from build123d import *

# Parameters (mm, degrees)
CYLINDER062_R       = 1.8
CYLINDER062_DEPTH   = 12
ARRAY001032_X_COUNT = 2
ARRAY001032_X_PITCH = 76
ARRAY001032_Y_COUNT = 2
ARRAY001032_Y_PITCH = 26
BOX036_W            = 4
BOX036_H            = 50
BOX036_DEPTH        = 10
FILLET018_R         = 1
ARRAY001038_X_COUNT = 2
ARRAY001038_X_PITCH = 58
CYLINDER064_R       = 3
CYLINDER064_DEPTH   = 12
ARRAY001034_X_COUNT = 2
ARRAY001034_X_PITCH = 76
ARRAY001034_Y_COUNT = 2
ARRAY001034_Y_PITCH = 26
CYLINDER063_R       = 5
CYLINDER063_DEPTH   = 10
ARRAY001033_X_COUNT = 2
ARRAY001033_X_PITCH = 76
ARRAY001033_Y_COUNT = 2
ARRAY001033_Y_PITCH = 26
CYLINDER066_R       = 1.8
CYLINDER066_DEPTH   = 50
ARRAY001036_Y_COUNT = 4
ARRAY001036_Y_PITCH = 6
BOX033_W            = 36
BOX033_H            = 25
BOX033_DEPTH        = 10
CYLINDER065_R       = 1.8
CYLINDER065_DEPTH   = 20
ARRAY001035_X_COUNT = 6
ARRAY001035_X_PITCH = 6
BOX032_W            = 40
BOX032_H            = 25
BOX032_DEPTH        = 10
BOX035_W            = 30
BOX035_H            = 50
BOX035_DEPTH        = 2
CYLINDER067_R       = 1.8
CYLINDER067_DEPTH   = 10
ARRAY001037_X_COUNT = 2
ARRAY001037_X_PITCH = 70
ARRAY001037_Y_COUNT = 2
ARRAY001037_Y_PITCH = 60
BOX034_W            = 80
BOX034_H            = 70
BOX034_DEPTH        = 2
FILLET017_R         = 4
BOX031_W            = 82
BOX031_H            = 32
BOX031_DEPTH        = 10
FILLET016_R         = 3
BOX029_W            = 86
BOX029_H            = 36
BOX029_DEPTH        = 10
FILLET015_R         = 3


with BuildPart() as obj1:
    # Cylinder062 → Cylinder062 (new body)
    with BuildSketch(Plane(origin=(5, 5, 0), x_dir=(1, 0, 0), z_dir=(0, 0, 1))):
        Circle(CYLINDER062_R)
    extrude(amount=CYLINDER062_DEPTH)

    # Array001032 X: obj1_2


with BuildPart() as obj1_1:
    add(obj1.part)
    with Locations(*[(i * ARRAY001032_X_PITCH, 0, 0) for i in range(1, ARRAY001032_X_COUNT)]):
        add(obj1.part)

    # Array001032 Y: obj1_2


with BuildPart() as obj1_2:
    add(obj1_1.part)
    with Locations(*[(0, i * ARRAY001032_Y_PITCH, 0) for i in range(1, ARRAY001032_Y_COUNT)]):
        add(obj1_1.part)


with BuildPart() as wire_hole_array:
    # Box036 → Box036 (new body)
    with BuildSketch(Plane(origin=(12, -7, 3), x_dir=(1, 0, 0), z_dir=(0, 0, 1))):
        with Locations((2, 25)):
            Rectangle(BOX036_W, BOX036_H)
    extrude(amount=BOX036_DEPTH)

    # Fillet018
    fillet018_edges = [wire_hole_array.edges().sort_by_distance(p)[0] for p in [
        (12, 18, 13),
        (12, 18, 3),
        (16, 18, 13),
        (16, 18, 3),
    ]]
    fillet(fillet018_edges, radius=FILLET018_R)

    # Array001038 X: wire hole array ×2


with BuildPart() as wire_hole_array_1:
    add(wire_hole_array.part)
    with Locations(*[(i * ARRAY001038_X_PITCH, 0, 0) for i in range(1, ARRAY001038_X_COUNT)]):
        add(wire_hole_array.part)


with BuildPart() as obj2:
    # Cylinder064 → Cylinder064 (new body)
    with BuildSketch(Plane(origin=(5, 5, -6), x_dir=(1, 0, 0), z_dir=(0, 0, 1))):
        Circle(CYLINDER064_R)
    extrude(amount=CYLINDER064_DEPTH)

    # Array001034 X: obj2_2


with BuildPart() as obj2_1:
    add(obj2.part)
    with Locations(*[(i * ARRAY001034_X_PITCH, 0, 0) for i in range(1, ARRAY001034_X_COUNT)]):
        add(obj2.part)

    # Array001034 Y: obj2_2


with BuildPart() as obj2_2:
    add(obj2_1.part)
    with Locations(*[(0, i * ARRAY001034_Y_PITCH, 0) for i in range(1, ARRAY001034_Y_COUNT)]):
        add(obj2_1.part)

    # Fusion043: union obj1, wire hole array
    add(obj1_2.part)
    add(wire_hole_array_1.part)


with BuildPart() as obj3:
    # Cylinder063 → Cylinder063 (new body)
    with BuildSketch(Plane(origin=(5, 5, 0), x_dir=(1, 0, 0), z_dir=(0, 0, 1))):
        Circle(CYLINDER063_R)
    extrude(amount=CYLINDER063_DEPTH)

    # Array001033 X: obj3_2


with BuildPart() as obj3_1:
    add(obj3.part)
    with Locations(*[(i * ARRAY001033_X_PITCH, 0, 0) for i in range(1, ARRAY001033_X_COUNT)]):
        add(obj3.part)

    # Array001033 Y: obj3_2


with BuildPart() as obj3_2:
    add(obj3_1.part)
    with Locations(*[(0, i * ARRAY001033_Y_PITCH, 0) for i in range(1, ARRAY001033_Y_COUNT)]):
        add(obj3_1.part)


with BuildPart() as led_hole_array001:
    # Cylinder066 → Cylinder066 (new body)
    with BuildSketch(Plane(origin=(19, 6, 6), x_dir=(0, 1, 0), z_dir=(1, 0, 0))):
        Circle(CYLINDER066_R)
    extrude(amount=CYLINDER066_DEPTH)

    # Array001036 Y: led hole array001 ×4


with BuildPart() as led_hole_array001_1:
    add(led_hole_array001.part)
    with Locations(*[(0, i * ARRAY001036_Y_PITCH, 0) for i in range(1, ARRAY001036_Y_COUNT)]):
        add(led_hole_array001.part)


with BuildPart() as led_wall_extraction:
    # Box033 → Box033 (new body)
    with BuildSketch(Plane(origin=(25, 1, 0), x_dir=(1, 0, 0), z_dir=(0, 0, 1))):
        with Locations((18, 12.5)):
            Rectangle(BOX033_W, BOX033_H)
    extrude(amount=BOX033_DEPTH)


with BuildPart() as led_hole_fusion:
    # Cylinder065 → Cylinder065 (new body)
    with BuildSketch(Plane(origin=(28, 37, 6), x_dir=(1, 0, 0), z_dir=(0, -1, 0))):
        Circle(CYLINDER065_R)
    extrude(amount=CYLINDER065_DEPTH)

    # Array001035 X: led hole fusion ×6


with BuildPart() as led_hole_fusion_1:
    add(led_hole_fusion.part)
    with Locations(*[(i * ARRAY001035_X_PITCH, 0, 0) for i in range(1, ARRAY001035_X_COUNT)]):
        add(led_hole_fusion.part)

    # Fusion044: union led hole array001, led wall extraction
    add(led_hole_array001_1.part)
    add(led_wall_extraction.part)


with BuildPart() as led_wall_cut:
    # Box032 → Box032 (new body)
    with BuildSketch(Plane(origin=(23, 3, 0), x_dir=(1, 0, 0), z_dir=(0, 0, 1))):
        with Locations((20, 12.5)):
            Rectangle(BOX032_W, BOX032_H)
    extrude(amount=BOX032_DEPTH)

    # Cut023008: cut led hole fusion
    add(led_hole_fusion_1.part, mode=Mode.SUBTRACT)


with BuildPart() as led_wall_cut_1:
    # Cut023008 placement: moved
    add(led_wall_cut.part.moved(Location((0, 0, 2))))


with BuildPart() as cube:
    # Box035 → Box035 (new body)
    with BuildSketch(Plane(origin=(58, 10, 0), x_dir=(1, 0, 0), z_dir=(0, 0, 1))):
        with Locations((15, 25)):
            Rectangle(BOX035_W, BOX035_H)
    extrude(amount=BOX035_DEPTH)


with BuildPart() as bottom_outer_hole_array:
    # Cylinder067 → Cylinder067 (new body)
    with BuildSketch(Plane(origin=(5, 5, 0), x_dir=(1, 0, 0), z_dir=(0, 0, 1))):
        Circle(CYLINDER067_R)
    extrude(amount=CYLINDER067_DEPTH)

    # Array001037 X: bottom outer hole array ×2


with BuildPart() as bottom_outer_hole_array_1:
    add(bottom_outer_hole_array.part)
    with Locations(*[(i * ARRAY001037_X_PITCH, 0, 0) for i in range(1, ARRAY001037_X_COUNT)]):
        add(bottom_outer_hole_array.part)

    # Array001037 Y: bottom outer hole array ×2


with BuildPart() as bottom_outer_hole_array_2:
    add(bottom_outer_hole_array_1.part)
    with Locations(*[(0, i * ARRAY001037_Y_PITCH, 0) for i in range(1, ARRAY001037_Y_COUNT)]):
        add(bottom_outer_hole_array_1.part)


with BuildPart() as bottom_outer_extraction_fusion:
    # Part__Mirroring001: instance of Cube
    add(cube.part.mirror(Plane(origin=(40, 0, 0), x_dir=(0, -1, 0), z_dir=(1, 0, 0))))

    # Fusion045: union Cube, bottom outer hole array
    add(cube.part)
    add(bottom_outer_hole_array_2.part)


with BuildPart() as bottom_outer_plate_fillet:
    # Box034 → Box034 (new body)
    with BuildSketch(Plane.XY):
        with Locations((40, 35)):
            Rectangle(BOX034_W, BOX034_H)
    extrude(amount=BOX034_DEPTH)

    # Cut023009: cut bottom outer extraction fusion
    add(bottom_outer_extraction_fusion.part, mode=Mode.SUBTRACT)


with BuildPart() as bottom_outer_plate_fillet_1:
    # Cut023009 placement: moved
    add(bottom_outer_plate_fillet.part.moved(Location((3, -17, 0))))

    # Fillet017
    fillet017_edges = [bottom_outer_plate_fillet_1.edges().sort_by_distance(p)[0] for p in [
        (3, -7, 1),
        (3, -17, 1),
        (83, -17, 1),
        (3, 43, 1),
        (3, 53, 1),
        (83, 53, 1),
        (83, 43, 1),
        (83, -7, 1),
    ]]
    fillet(fillet017_edges, radius=FILLET017_R)


with BuildPart() as obj4:
    # Box031 → Box031 (new body)
    with BuildSketch(Plane(origin=(2, 2, 2), x_dir=(1, 0, 0), z_dir=(0, 0, 1))):
        with Locations((41, 16)):
            Rectangle(BOX031_W, BOX031_H)
    extrude(amount=BOX031_DEPTH)

    # Fillet016
    fillet016_edges = [obj4.edges().sort_by_distance(p)[0] for p in [
        (2, 2, 7),
        (2, 34, 7),
        (84, 2, 7),
        (84, 34, 7),
    ]]
    fillet(fillet016_edges, radius=FILLET016_R)


with BuildPart() as obj5:
    # Box029 → Box029 (new body)
    with BuildSketch(Plane.XY):
        with Locations((43, 18)):
            Rectangle(BOX029_W, BOX029_H)
    extrude(amount=BOX029_DEPTH)

    # Fillet015
    fillet015_edges = [obj5.edges().sort_by_distance(p)[0] for p in [
        (0, 0, 5),
        (0, 36, 5),
        (86, 0, 5),
        (86, 36, 5),
    ]]
    fillet(fillet015_edges, radius=FILLET015_R)

    # Cut023006: cut obj4
    add(obj4.part, mode=Mode.SUBTRACT)

    # Fusion042: union obj3, led wall cut, bottom outer plate fillet
    add(obj3_2.part)
    add(led_wall_cut_1.part)
    add(bottom_outer_plate_fillet_1.part)

    # Cut023007: cut obj2
    add(obj2_2.part, mode=Mode.SUBTRACT)


solid = obj5.part
Build history of the part. All positions in model axes, mm. A direction names the side the tool comes from. Round coordinates to 2 decimals unless told otherwise and drop trailing zeros. Write each loop counter-clockwise with the first axis right and the second up, starting at its lowest first coordinate (ties: lowest second). Pieces come first, ordered by that corner, then holes. Notation, with made-up numbers: M 82,87.5 L 94,87.5 A24 cw 94,97.5 Z; hole C -24.75,52 d5. An arc over 180 degrees is marked long. Answer as a JSON object with one key per item and string values. Group by question number.
(1) Drill centre lines: L1, parallel to Y at x = 42, z = 3; L2, parallel to X at y = 5, z = 3.6; L3, parallel to X at y = 5, z = 7.25. Where is each one in solid material? Low to high.
(2) Flat gauge pins, fed straight in: pin 1 (4 mm diameter, centred on x = 78, y = 48, fed in from +Z); pin 2 (2 mm diameter, centred on x = 62.5, z = 9.5, fed in from -Y); pin 3 (3 mm diameter, centred on x = 28, z = 8, fed in from +Y); pin 4 (12 mm diameter, centred on x = 14.5, y = -1.5, fed in from -Z). Where does each tip first touch, or does it go through?
(3) Cut at D-D (z = 8). Give the number of separate pieces and of enclosed holes in the cut face, and give its area (3 significant figures).
(4) Mould opens along Y. For faces 1 (the flat face through (86, 18, 5)), 2 (the cylindrical face through (76.572, -13.095, 0.986)), 3 (the cylindrical face through (0.86, 0.9, 5.07)) say: pulls with the +Y half, pulls with the -Y half, needs draft (parallel to the pull), parting line crosses it, or undercut.
(5) Cut at A-A (x = 72). Give the cut face in (y, z).
(6) Cut at C-C (y = 18). Give the cut face in (x, z).
(7) Which spindle directions (+Z, -Z, +X, -X, +Y, -Y) get a long thin tool onto all of the face, cutting with end or side? Do faces 4 (the flat face through (74, 35, 7)), 5 (the cylindrical face through (35.663, 27.014, 7.311)), 6 (the flat face through (3, -12, 1)). Say none if no direction does.
(8) Cut at B-B (x = 58). Give the cut face in (y, z).
Responses:
{
 "1": {"L1": "y = 0 to 2, 26 to 28, 34 to 36", "L2": "x = 0 to 2, 8 to 10, 23 to 25, 61 to 63, 76 to 78, 84 to 86", "L3": "x = 0 to 3.2, 6.8 to 10, 76 to 79.2, 82.8 to 86"},
 "2": {"pin 1": "stops at z = 2", "pin 2": "stops at y = 0", "pin 3": "stops at y = 36", "pin 4": "stops at z = 0"},
 "3": {"separate pieces": "19", "enclosed holes": "4", "area": "690 mm2"},
 "4": {"face 1": "needs draft", "face 2": "undercut", "face 3": "pulls with the -Y half"},
 "5": {"outline": "M -17,0 L -7,0 L -7,2 L -17,2 Z; M 0,0 L 36,0 L 36,3 L 34,3 L 34,2 L 2,2 L 2,3 L 0,3 Z; M 43,0 L 53,0 L 53,2 L 43,2 Z"},
 "6": {"outline": "M 0,0 L 86,0 L 86,10 L 84,10 L 84,2 L 63,2 L 63,6.2 L 61,6.2 L 61,2 L 25,2 L 25,6.2 L 23,6.2 L 23,2 L 2,2 L 2,10 L 0,10 Z; M 23,9.8 L 25,9.8 L 25,12 L 23,12 Z; M 61,9.8 L 63,9.8 L 63,12 L 61,12 Z"},
 "7": {"face 4": "+Z, +Y, -Y", "face 5": "none", "face 6": "+Z, -Z, -X, -Y"},
 "8": {"outline": "M -17,0 L 53,0 L 53,2 L 36,2 L 36,10 L 34,10 L 34,2 L 28,2 L 28,6.2 L 26,6.2 L 26,2 L 2,2 L 2,10 L 0,10 L 0,2 L -17,2 Z; M 26,9.8 L 28,9.8 L 28,12 L 26,12 Z"}
}
